Geometry check sheet. Reference: the model listing, model coordinates, mm. A direction names the side the tool comes from. Give positions to 0.01 mm unless a question says otherwise; leave off trailing zeros. Write each loop counter-clockwise with the first axis right and the second up, starting at its lowest first coordinate (ties: lowest second). Pieces come first, ordered by that corner, then holes. Notation, with made-up numbers: (-16, 61.25) -> (41, 61.25) arc R26 cw to (41, 79.25) -> close; hole circle Ø5 at (10.5, -35.75). An arc over 180 degrees is marked (long way). One line per item, written item: value.
from build123d import *

# Parameters (mm, degrees)
SKETCH005_W             = 6.1
SKETCH005_H             = 5.1
PAD005_DEPTH            = 12.3
SKETCH006_R             = 2.55
SKETCH006_R_2           = 1.8
PAD006_DEPTH            = 2
SKETCH007_W             = 1
SKETCH007_H             = 6
PAD007_DEPTH            = 3
BODY002_PLACEMENT_ANGLE = 90


with BuildPart() as part:
    # Sketch005 → Pad005 (new body)
    with BuildSketch(Plane.XZ):
        Rectangle(SKETCH005_W, SKETCH005_H)
    extrude(amount=-PAD005_DEPTH)

    # Sketch006 → Pad006 (join)
    with BuildSketch(Plane.XZ):
        Circle(SKETCH006_R)
        with Locations((-0.041022, 0)):
            Circle(SKETCH006_R_2, mode=Mode.SUBTRACT)
    extrude(amount=PAD006_DEPTH)

    # Sketch007 → Pad007 (join, symmetric)
    with BuildSketch(Plane.YZ):
        with Locations((1.5, -3)):
            Rectangle(SKETCH007_W, SKETCH007_H)
        with Locations((11.5, -3)):
            Rectangle(SKETCH007_W, SKETCH007_H)
    extrude(amount=PAD007_DEPTH, both=True)


with BuildPart() as part_1:
    # Body002 placement: moved
    add(part.part.moved(Location((7, 5, 4.5))).rotate(Axis((7, 5, 4.5), (0, 0, 1)), BODY002_PLACEMENT_ANGLE))


solid = part_1.part
1) Tool access check on faces 4 (the flat face through (7, 7.8, 4.5)), 5 (the flat face through (-5, 5, 0)), 6 (the flat face through (7, 5, 5)), 7 (the flat face through (5.5, 2, 0.2)), 8 (the flat face through (5.5, 8, 0.2)). Record the directions out of +Z, -Z, +X, -X, +Y, -Y that give a thin tool (end or side, any length) a straight path to the whole face; none if there is none.
Verdict:
face 4: +X, +Y
face 5: -Z, -X, +Y, -Y
face 6: +X
face 7: -Z, +X, -X, -Y
face 8: -Z, +X, -X, +Y
2) Sectioned sample at D-D on z = 6.75. Record the cut outline in (x, y).
Verdict:
outline: (-5.3, 1.95) -> (7, 1.95) -> (7, 3.8) -> (9, 3.8) -> (9, 6.2) -> (7, 6.2) -> (7, 8.05) -> (-5.3, 8.05) -> close
3) Sectioned sample at B-B on x = 7.75. Record the cut outline in (y, z).
Verdict:
outline: circle Ø5.1 at (5, 4.5); hole circle Ø3.6 at (4.96, 4.5)
4) Sectioned sample at C-C on y = 7. Record the cut outline in (x, z), plus the area to 3 significant figures.
Verdict:
outline: (-5.3, 1.95) -> (-5, 1.95) -> (-5, -1.5) -> (-4, -1.5) -> (-4, 1.95) -> (5, 1.95) -> (5, -1.5) -> (6, -1.5) -> (6, 1.95) -> (7, 1.95) -> (7, 2.92) -> (9, 2.92) -> (9, 6.08) -> (7, 6.08) -> (7, 7.05) -> (-5.3, 7.05) -> close
area: 76.0 mm^2
5) Sectioned sample at A-A on z = 4.5. Record the cut outline in (x, y).
Verdict:
outline: (-5.3, 1.95) -> (7, 1.95) -> (7, 2.45) -> (9, 2.45) -> (9, 3.16) -> (7, 3.16) -> (7, 6.76) -> (9, 6.76) -> (9, 7.55) -> (7, 7.55) -> (7, 8.05) -> (-5.3, 8.05) -> close
6) Scan lines: probe 1 along X at (y, z) = (5.5, 0); probe 2 along Z at (x, y) = (4, 7.5); probe 3 along X at (y, z) = (5.5, 4.5). Record each from-to range of solid material in increasing order.
Verdict:
probe 1: -5 to -4, 5 to 6
probe 2: 1.95 to 7.05
probe 3: -5.3 to 7
7) Depth check by flat-ended pin: pin 1 Ø3 at (y, z) = (3.5, 0) entering from -X; pin 2 Ø0.5 at (x, z) = (-4.5, -0.5) entering from +Y; pin 3 Ø3 at (y, z) = (5, -0.5) entering from +X. Enter the tip coordinate at first touch or a pass-through.
Verdict:
pin 1: x = -5
pin 2: y = 8
pin 3: x = 6
8) Mould release check, pull along X, two halves, no side actions. Record for faces 1 (the flat face through (5, 5, 0)), 2 (the flat face through (-4.5, 5, -1.5)), 3 (the flat face through (6, 5, 0)): released by +X, released by -X, zero draft, split by the parting line, or undercut.
Verdict:
face 1: undercut
face 2: zero draft
face 3: released by +X
